The model under review builds one solid part; all positions refer to its coordinate system, in mm. Give positions to 0.01 mm unless a question says otherwise; leave off trailing zeros. Order: outer loops, then holes, each group sorted by start corner. A loop starts at its lowest first (then second) coordinate and runs counter-clockwise, first axis right, second up. Notation, with made-up numbers: (-15, -12) - (29, -12) arc R18 ccw to (29, 3) - close; hole circle Ø7 at (48, 16.5). An arc over 180 degrees is marked (long way). Use CSV: the item, a comma, the result in double quotes. Start each with the question number.
```python
from build123d import *

# Parameters (mm, degrees)
F1_R     = 14.5
F2_DEPTH = 8
F4_DEPTH = 5.5
F5_R     = 5


with BuildPart() as f2:
    # F1 (on Top) → F2 (new body, symmetric)
    with BuildSketch(Plane.XY):
        Circle(F1_R)
    extrude(amount=F2_DEPTH, both=True)

    # F3 (on Top) → F4 (cut, symmetric)
    with BuildSketch(Plane.XY):
        Polygon((-11.1578674376, 0), (-5.6730398803, -9.5), (5.2966152343, -9.5), (10.7814427916, 0), (5.2966152343, 9.5), (-5.6730398803, 9.5), align=None)
    extrude(amount=F4_DEPTH, both=True, mode=Mode.SUBTRACT)

    # F5
    f5_edges = [f2.edges().sort_by_distance(p)[0] for p in [
        (-14.5, 0, 8),
        (-14.5, 0, -8),
    ]]
    fillet(f5_edges, radius=F5_R)


solid = f2.part
```
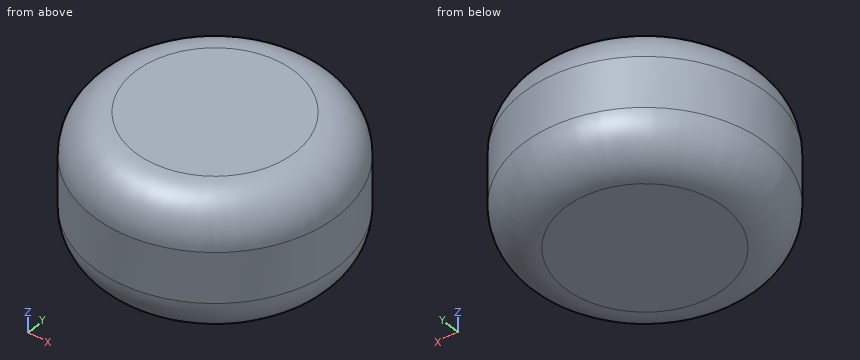
1. To check wall thickness, follow L1, parallel to Z at x = 9.25, y = -0.75; L2, parallel to Y at x = 0, z = 2.75; L3, parallel to X at y = -9, z = -3.5. State the ranges of each line that lie inside material, in increasing order. Write a range as [from, to].
2. Consider section A-A (x = 0). Give the boundary of the cut face in (y, z), and give its area (3 significant figures).
3. Consider section B-B (z = 3.75). Give the boundary of the cut face in (x, y).
4. Consider section C-C (z = -6). Give the boundary of the cut face in (x, y), and give its area (3 significant figures).
5. Clearance check with flat-ended pins moving along their axes: pin 1 (2 mm diameter, centred on x = -10, z = -0.5, fed in from +Y); pin 2 (3.5 mm diameter, centred on x = 1, z = -1.5, fed in from -Y); pin 3 (3 mm diameter, centred on x = 11, y = 10, fed in from -Z). State where each tip first meets the part, or that it passes through.
Answers follow:
1,L1,"z = [-8, -5.5], [5.5, 8]"
1,L2,"y = [-14.5, -9.5], [9.5, 14.5]"
1,L3,"x = [-11.34, -5.96], [5.59, 11.34]"
2,outline,"(-14.5, -3) arc R5 ccw to (-9.5, -8) - (9.5, -8) arc R5 ccw to (14.5, -3) - (14.5, 3) arc R5 ccw to (9.5, 8) - (-9.5, 8) arc R5 ccw to (-14.5, 3) - close; hole (-9.5, -5.5) - (9.5, -5.5) - (9.5, 5.5) - (-9.5, 5.5) - close"
2,area,"234 mm^2"
3,outline,"circle Ø28.89 at (0, 0); hole (-11.16, 0) - (-5.67, -9.5) - (5.3, -9.5) - (10.78, 0) - (5.3, 9.5) - (-5.67, 9.5) - close"
4,outline,"circle Ø27 at (0, 0)"
4,area,"573 mm^2"
5,pin 1,"stops at y = 11.37"
5,pin 2,"stops at y = -14.5"
5,pin 3,"stops at z = -6.17"
